Geometry: see drawing. Coordinates: mm, zero at the bounding-box minimum. A direction names the side the tool comes from. Give positions to 0.01 mm unless a question says otherwise; leave off trailing zeros. Loops run counter-clockwise (first coordinate to the right, second up) from the corner with the lowest first, then second, coordinate; pieces in that order, holes last. Notation, with made-up numbers: (64, -4) - (74, -4) arc R30 cw to (74, 33) - close; hole circle Ø9 at (-30.5, 67.5). An arc over 180 degrees is marked (long way). Use one line per item in the form item = value.
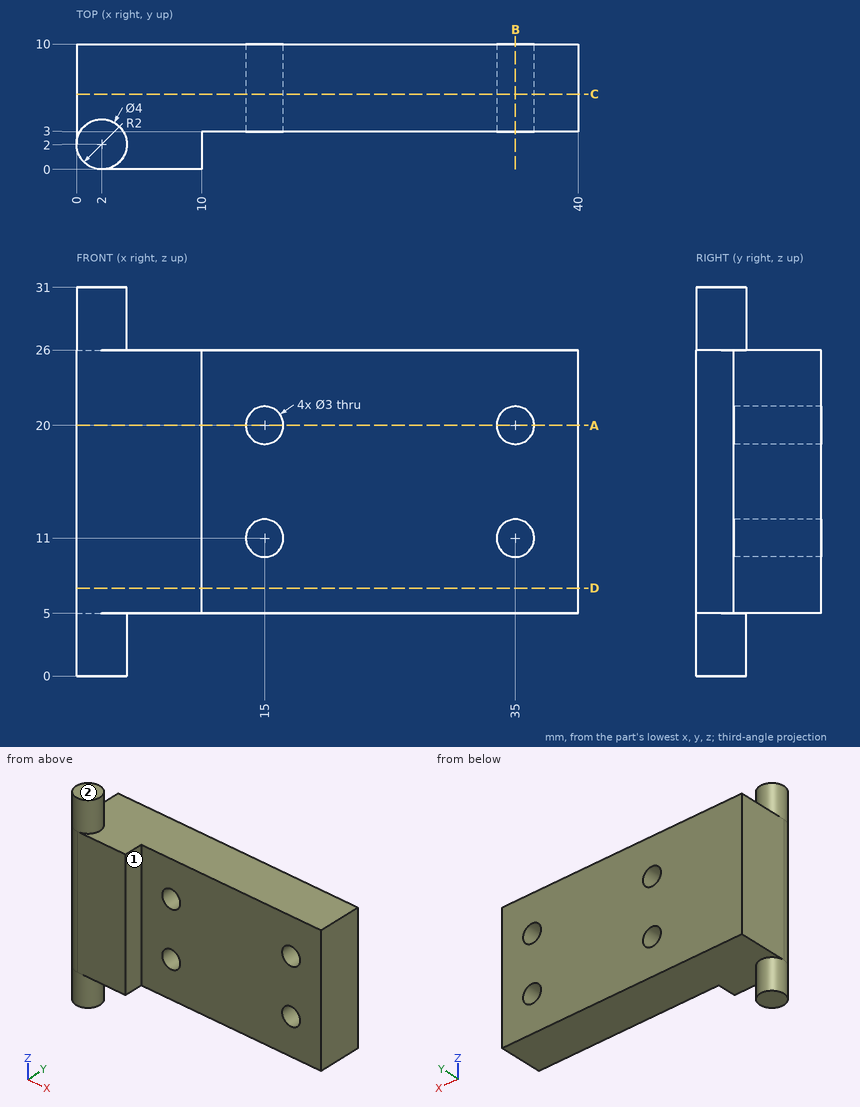
(1) Access query for the marked faces 1 and 2. Directions: +Z, -Z, +X, -X, +Y, -Y. A direction counts if a zero-diameter tool reaches every point of the face in a straight line with its end or side. Return the directions, or none.
Solution:
face_1 = +Z, -Z, +X, -Y
face_2 = +Z, +X, -X, +Y, -Y
(2) Material intervals for L1, parallel to Z at x = 35, y = 6; L2, parallel to Z at x = 14, y = 3.5; L3, parallel to Y at x = 10.5, z = 17.5, sorted ascending. Write a range as from..to.
Solution:
L1 = 5..9.5, 12.5..18.5, 21.5..26
L2 = 5..9.88, 12.12..18.88, 21.12..26
L3 = 3..10
(3) Cut plane C-C (y = 6). Return the cut outline in (x, z), plus the area to 3 significant figures.
Solution:
outline = (0, 5) - (40, 5) - (40, 26) - (0, 26) - close; hole circle Ø3 at (15, 11); hole circle Ø3 at (15, 20); hole circle Ø3 at (35, 11); hole circle Ø3 at (35, 20)
area = 812 mm2
(4) Pin query (flat end, axial travel): P1, Ø1.5, axis at x = 11, y = 3, coming from the +Z side; P2, Ø6, axis at x = 13.5, z = 15, coming from the -Y side; P3, Ø1.5, axis at x = 22, y = 7.5, coming from the -Z side; P4, Ø2.5, axis at x = 15, z = 20, coming from the -Y side. Return the tip coordinate at first contact, or that it passes through.
Solution:
P1 = 26
P2 = 3
P3 = 5
P4 = through
(5) Cut plane A-A (z = 20). Return the cut outline in (x, y), plus the area to 3 significant figures.
Solution:
outline = (0, 2) arc R2 ccw to (2, 0) - (10, 0) - (10, 3) - (13.5, 3) - (13.5, 10) - (0, 10) - close; (16.5, 3) - (33.5, 3) - (33.5, 10) - (16.5, 10) - close; (36.5, 3) - (40, 3) - (40, 10) - (36.5, 10) - close
area = 267 mm2
(6) Cut plane D-D (z = 7). Return the cut outline in (x, y), plus the area to 3 significant figures.
Solution:
outline = (0, 2) arc R2 ccw to (2, 0) - (10, 0) - (10, 3) - (40, 3) - (40, 10) - (0, 10) - close
area = 309 mm2
(7) Cut plane B-B (x = 35). Return the cut outline in (y, z), plus the area to 3 significant figures.
Solution:
outline = (3, 5) - (10, 5) - (10, 9.5) - (3, 9.5) - close; (3, 12.5) - (10, 12.5) - (10, 18.5) - (3, 18.5) - close; (3, 21.5) - (10, 21.5) - (10, 26) - (3, 26) - close
area = 105 mm2
